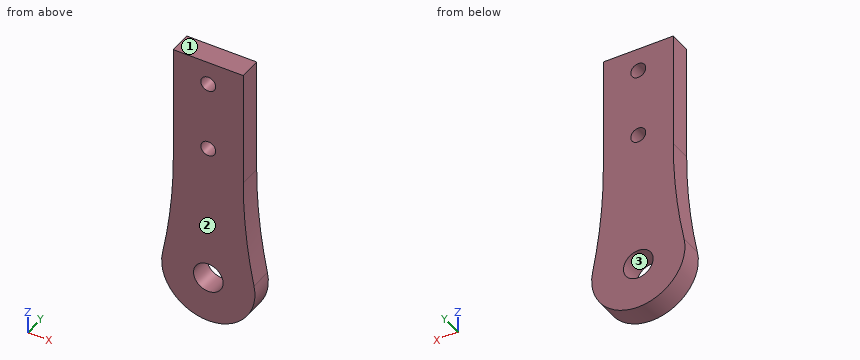
from build123d import *

# Parameters (mm, degrees)
SKETCH1_R           = 3.175
SKETCH1_R_2         = 1.6
BOSS_EXTRUDE1_DEPTH = 4.7625


with BuildPart() as part:
    # Sketch1 → Boss-Extrude1 (new body)
    with BuildSketch(Plane(origin=(0, 0, 0), x_dir=(1, 0, 0), z_dir=(0, 1, 0))):
        with BuildLine():
            Line((-7.5, 0), (7.5, 0))
            Line((7.5, 0), (7.5, 25))
            ThreePointArc((7.5, 25), (8.076926638, 36.567307336), (9.801980198, 48.01980198))
            ThreePointArc((9.801980198, 48.01980198), (0, 60), (-9.801980198, 48.01980198))
            ThreePointArc((-9.801980198, 48.01980198), (-8.076926638, 36.567307336), (-7.5, 25))
            Line((-7.5, 25), (-7.5, 0))
        make_face()
        with Locations((0, 50)):
            Circle(SKETCH1_R, mode=Mode.SUBTRACT)
        with Locations((0, 5)):
            Circle(SKETCH1_R_2, mode=Mode.SUBTRACT)
        with Locations((0, 20)):
            Circle(SKETCH1_R_2, mode=Mode.SUBTRACT)
    extrude(amount=BOSS_EXTRUDE1_DEPTH)


solid = part.part
Can you work these out from the model? Positions are in its coordinate system, mm. Face numbers are marked on the shaded views. Coordinates: 2 decimals unless noted, no trailing zeros. Order: outer loops, then holes, each group sorted by start corner. A loop starts at its lowest first (then second) coordinate and runs counter-clockwise, first axis right, second up. Notation, with made-up numbers: (66, 5.25) - (95, 5.25) arc R9 cw to (95, 15.25) - close; hole circle Ø8 at (17, 42.5). An arc over 180 degrees is marked (long way). Answer as a JSON object with one key per item and string values. Group by question number.
Q1. Imagine slicing it at D-D (z = -50). Please give me the cut outline in (x, y) (1 decimal).
Q2. Imagine slicing it at A-A (x = 0). Please give me the cut outline in (y, z) (1 decimal), and give its area (3 significant figures).
Q3. Will these pins go through, and if not, where does the flat tip stop? P1, Ø3.5, axis at x = 0, z = -5, coming from the -Y side; P2, Ø1.5, axis at y = 2, z = -30.5, coming from the -X side; P3, Ø1, axis at y = 4, z = -27.5, coming from the +X side; P4, Ø2.5, axis at y = 3.5, z = -10.5, coming from the -X side.
Q4. We'd pull the mould along Z, two halves only. Please class the marked faces 1, 2 and 3: +Z half, -Z half, draft (parallel to the pull), parting line (faces both ways), or undercut.
Q5. Imagine slicing it at B-B (z = -5). Please give me the cut outline in (x, y), and give its area (3 significant figures).
Q6. I need wall thicknesses on line 1 (Z direction, x = 0, y = 3.45) (3 decimals); line 2 (X direction, y = 3.6, z = -20); line 3 (Z direction, x = -0.5, y = 0.2). Which ranges of each line are inside material? Lowest first, please. Write a range as from..to.
Q7. Imagine slicing it at C-C (y = 2.1). Please give me the cut outline in (x, z) (3 decimals), and give its area (3 significant figures).
Determined:
{
 "1": {"outline": "(-10, 0) - (-3.2, 0) - (-3.2, 4.8) - (-10, 4.8) - close; (3.2, 0) - (10, 0) - (10, 4.8) - (3.2, 4.8) - close"},
 "2": {"outline": "(0, -60) - (4.8, -60) - (4.8, -53.2) - (0, -53.2) - close; (0, -46.8) - (4.8, -46.8) - (4.8, -21.6) - (0, -21.6) - close; (0, -18.4) - (4.8, -18.4) - (4.8, -6.6) - (0, -6.6) - close; (0, -3.4) - (4.8, -3.4) - (4.8, 0) - (0, 0) - close", "area": "225 mm2"},
 "3": {"P1": "stops at y = 0", "P2": "stops at x = -7.67", "P3": "stops at x = 7.54", "P4": "stops at x = -7.5"},
 "4": {"face 1": "+Z half", "face 2": "draft", "face 3": "undercut"},
 "5": {"outline": "(-7.5, 0) - (-1.6, 0) - (-1.6, 4.76) - (-7.5, 4.76) - close; (1.6, 0) - (7.5, 0) - (7.5, 4.76) - (1.6, 4.76) - close", "area": "56.2 mm2"},
 "6": {"line 1": "z = -60..-53.175, -46.825..-21.6, -18.4..-6.6, -3.4..0", "line 2": "x = -7.5..-1.6, 1.6..7.5", "line 3": "z = -59.99..-53.14, -46.86..-21.52, -18.48..-6.52, -3.48..0"},
 "7": {"outline": "(-9.802, -48.02) arc R10 ccw (long way) to (9.802, -48.02) arc R116.25 cw to (7.5, -25) - (7.5, 0) - (-7.5, 0) - (-7.5, -25) arc R116.25 cw to start; hole circle Ø6.35 at (0, -50); hole circle Ø3.2 at (0, -20); hole circle Ø3.2 at (0, -5)", "area": "904 mm2"}
}
